from build123d import *
from build123d.topology import SkipClean

# Parameters (mm, degrees)
BOSS_EXTRUDE1_DEPTH = 2
BOSS_EXTRUDE2_START = 3
BOSS_EXTRUDE2_DEPTH = 3
CUT_EXTRUDE1_REACH  = 22.009
SKETCH5_R           = 7.5
BOSS_EXTRUDE3_DEPTH = 1
SKETCH8_W           = 3
SKETCH8_H           = 5
BOSS_EXTRUDE4_DEPTH = 39
BOSS_EXTRUDE5_DEPTH = 2
CUT_EXTRUDE2_REACH  = 72.907
SKETCH10_R          = 3.5
CUT_EXTRUDE4_REACH  = 45.872
SKETCH11_R          = 0.9
BOSS_EXTRUDE6_DEPTH = 7.7
SKETCH16_W          = 2
SKETCH16_H          = 3
BOSS_EXTRUDE7_DEPTH = 14.7


with BuildPart() as part:
    # Sketch2 → Boss-Extrude1 (new body)
    with BuildSketch(Plane.XY):
        with BuildLine():
            ThreePointArc((13.7, 0), (9.687362902, 9.687362902), (0, 13.7))
            ThreePointArc((0, 13.7), (-9.687362902, 9.687362902), (-13.7, 0))
            Line((-13.7, 0), (13.7, 0))
        make_face()
        with BuildLine():
            Line((13.7, 0), (-13.7, 0))
            ThreePointArc((-13.7, 0), (0, -13.7), (13.7, 0))
        make_face()
        with BuildLine():
            Line((13.7, 13.7), (0, 13.7))
            ThreePointArc((0, 13.7), (9.687362902, 9.687362902), (13.7, 0))
            Line((13.7, 0), (13.7, 13.7))
        make_face()
        with BuildLine():
            Line((0, 13.7), (-13.7, 13.7))
            Line((-13.7, 13.7), (-13.7, 0))
            ThreePointArc((-13.7, 0), (-9.687362902, 9.687362902), (0, 13.7))
        make_face()
        with BuildLine():
            ThreePointArc((13.7, 0), (9.687362902, 9.687362902), (0, 13.7))
            ThreePointArc((0, 13.7), (-9.687362902, 9.687362902), (-13.7, 0))
            Line((-13.7, 0), (13.7, 0))
        make_face()
        with BuildLine():
            Line((13.7, 0), (-13.7, 0))
            ThreePointArc((-13.7, 0), (0, -13.7), (13.7, 0))
        make_face()
    extrude(amount=BOSS_EXTRUDE1_DEPTH)

    # Sketch3 → Boss-Extrude2 (add)
    with SkipClean():  # the faces are left unmerged after this step: merging them gives an invalid solid
        with BuildSketch(Plane(origin=(0, 0, 0), x_dir=(-1, 0, 0), z_dir=(0, 0, -1)).offset(BOSS_EXTRUDE2_START)):
            with BuildLine():
                Line((-11.7, 0), (-13.7, 0))
                ThreePointArc((-13.7, 0), (-13.491866216, -2.378980034), (-12.873788905, -4.685675964))
                Line((-12.873788905, -4.685675964), (-10.994403663, -4.001635677))
                ThreePointArc((-10.994403663, -4.001635677), (-11.52225071, -2.031683679), (-11.7, 0))
            make_face()
            with BuildLine():
                ThreePointArc((11.7, 0), (11.52225071, -2.031683679), (10.994403663, -4.001635677))
                Line((10.994403663, -4.001635677), (12.873788905, -4.685675964))
                ThreePointArc((12.873788905, -4.685675964), (13.491866216, -2.378980034), (13.7, 0))
                Line((13.7, 0), (11.7, 0))
            make_face()
        extrude(amount=-BOSS_EXTRUDE2_DEPTH)

    # Sketch5 → Cut-Extrude1 (cut, up to next)
    with BuildSketch(Plane.XY.offset(2), mode=Mode.PRIVATE) as cut_extrude1_sk1:
        Circle(SKETCH5_R)
    cut_extrude1_tool1 = extrude(cut_extrude1_sk1.sketch, amount=-CUT_EXTRUDE1_REACH, mode=Mode.PRIVATE) & part.part
    add(cut_extrude1_tool1.solids().sort_by_distance((0, 0, 2))[0], mode=Mode.SUBTRACT)

    # Sketch7 → Boss-Extrude3 (add)
    with SkipClean():  # the faces are left unmerged after this step: merging them gives an invalid solid
        with BuildSketch(Plane(origin=(0, 13.7, 0), x_dir=(1, 0, 0), z_dir=(0, 1, 0))):
            Polygon((0, 0), (13.7, 0), (0, 27), (-13.7, 0), align=None)
            Polygon((13.7, -2), (13.7, 0), (0, 0), (-13.7, 0), (-13.7, -2), align=None)
        extrude(amount=BOSS_EXTRUDE3_DEPTH)

    # Sketch8 → Boss-Extrude4 (add)
    with SkipClean():  # the faces are left unmerged after this step: merging them gives an invalid solid
        with BuildSketch(Plane.XY.offset(2)):
            with Locations((-12.2, 4.5)):
                Rectangle(SKETCH8_W, SKETCH8_H)
            with Locations((12.2, 4.5)):
                Rectangle(SKETCH8_W, SKETCH8_H)
        extrude(amount=BOSS_EXTRUDE4_DEPTH)

    # Sketch9 → Boss-Extrude5 (add)
    with SkipClean():  # the faces are left unmerged after this step: merging them gives an invalid solid
        with BuildSketch(Plane.XY.offset(41)):
            Polygon((-10.7, 2), (-13.7, 2), (0, -8.786353055), (13.7, 2), (10.7, 2), (10.7, 7), (-10.7, 7), align=None)
        extrude(amount=-BOSS_EXTRUDE5_DEPTH)

    # Sketch10 → Cut-Extrude2 (cut, up to next)
    with BuildSketch(Plane.XY.offset(41), mode=Mode.PRIVATE) as cut_extrude2_sk1:
        Circle(SKETCH10_R)
    cut_extrude2_tool1 = extrude(cut_extrude2_sk1.sketch, amount=-CUT_EXTRUDE2_REACH, mode=Mode.PRIVATE) & part.part
    add(cut_extrude2_tool1.solids().sort_by_distance((0, 0, 41))[0], mode=Mode.SUBTRACT)

    # Sketch11 → Cut-Extrude4 (cut, up to next)
    with BuildSketch(Plane.XY.offset(2), mode=Mode.PRIVATE) as cut_extrude4_sk1:
        with Locations((0, 10)):
            Circle(SKETCH11_R)
    cut_extrude4_tool1 = extrude(cut_extrude4_sk1.sketch, amount=-CUT_EXTRUDE4_REACH, mode=Mode.PRIVATE) & part.part
    # Sketch11 → Cut-Extrude4 (cut, up to next)
    with BuildSketch(Plane.XY.offset(2), mode=Mode.PRIVATE) as cut_extrude4_sk2:
        with Locations((0, -10)):
            Circle(SKETCH11_R)
    cut_extrude4_tool2 = extrude(cut_extrude4_sk2.sketch, amount=-CUT_EXTRUDE4_REACH, mode=Mode.PRIVATE) & part.part
    add(cut_extrude4_tool1.solids().sort_by_distance((0, 10, 2))[0], mode=Mode.SUBTRACT)
    add(cut_extrude4_tool2.solids().sort_by_distance((0, -10, 2))[0], mode=Mode.SUBTRACT)

    # Sketch15 → Boss-Extrude6 (add, through all)
    with SkipClean():  # the faces are left unmerged after this step: merging them gives an invalid solid
        with BuildSketch(Plane(origin=(0, 7, 0), x_dir=(1, 0, 0), z_dir=(0, 1, 0))):
            Polygon((-10.7, -2), (-13.7, -2), (-13.7, -41), (13.7, -41), (13.7, -2), (10.7, -2), (10.7, -39), (-10.7, -39), align=None)
        extrude(amount=BOSS_EXTRUDE6_DEPTH)

    # Sketch16 → Boss-Extrude7 (add, through all)
    with SkipClean():  # the faces are left unmerged after this step: merging them gives an invalid solid
        with BuildSketch(Plane(origin=(0, 0, 0), x_dir=(1, 0, 0), z_dir=(0, 1, 0))):
            with Locations((12.7, 1.5)):
                Rectangle(SKETCH16_W, SKETCH16_H)
            with Locations((-12.7, 1.5)):
                Rectangle(SKETCH16_W, SKETCH16_H)
        extrude(amount=BOSS_EXTRUDE7_DEPTH)


solid = part.part
Input: part model. Units: mm. Frame: model coordinates. A direction names the side the tool comes from. Round coordinates to 2 decimals unless told otherwise and drop trailing zeros. Loops run counter-clockwise (first coordinate to the right, second up) from the corner with the lowest first, then second, coordinate; pieces in that order, holes last. Notation, with made-up numbers: (80.5, 53.25) -> (118.5, 53.25) arc R17 ccw to (118.5, 63.25) -> close; hole circle Ø5 at (-32, -5). An arc over 180 degrees is marked (long way). Answer as a JSON object with one key per item and string values. Group by question number.
1) Section query B-B on z = 1. Output: boundary loops of the cut face in (x, y).
2) Ray query, L1, parallel to Y at x = 0, z = 1.65; L2, parallel to Z at x = 9.25, y = 7.25; L3, parallel to X at y = 2.25, z = 24. Return the intervals inside material, ascending.
3) Section query C-C on y = 10. Output: boundary loops of the cut face in (x, z), plus the area to 3 significant figures.
4) Section query A-A on z = 21.5. Output: boundary loops of the cut face in (x, y).
5) Section query D-D on x = 5.25. Output: boundary loops of the cut face in (y, z).
6) Draft query along Z for faces 1 (the cylindrical face through (-7.493, 0.33, 1.014)), 2 (the flat face through (-10.7, 8, 20)), 3 (the flat face through (6.174, 14.193, -14.832)). Return one class per face: +Z half, -Z half, draft (parallel to the pull), parting line (faces both ways), or undercut.
7) Reachability of faces 4 (the flat face through (10.7, 8, 20)), 5 (the flat face through (12, 2, 20)), 6 (the flat face through (-11.7, 7, -1)) from +Z, -Z, +X, -X, +Y, -Y: full face, straight path, thin tool, end or side. Return the list, or none.
8) Pin query (flat end, axial travel): pin 1 (4 mm diameter, centred on x = -4.5, y = 0, fed in from -Z); pin 2 (1.4 mm diameter, centred on x = -12, y = 6, fed in from -Z); pin 3 (3.5 mm diameter, centred on x = -12, z = 12, fed in from -Y). Return the tip coordinate at first contact, or that it passes through.
Reply:
{
 "1": {"outline": "(-13.7, 0) arc R13.7 ccw to (13.7, 0) -> (13.7, 14.7) -> (-13.7, 14.7) -> close; hole circle Ø15 at (0, 0); hole circle Ø1.8 at (0, -10); hole circle Ø1.8 at (0, 10)"},
 "2": {"L1": "y = -13.7 to -10.9, -9.1 to -7.5, 7.5 to 9.1, 10.9 to 14.7", "L2": "z = 0 to 2, 39 to 41", "L3": "x = -13.7 to -10.7, 10.7 to 13.7"},
 "3": {"outline": "(-13.7, -3) -> (-11.7, -3) -> (-11.7, 0) -> (-0.9, 0) -> (-0.9, 2) -> (-10.7, 2) -> (-10.7, 39) -> (10.7, 39) -> (10.7, 2) -> (0.9, 2) -> (0.9, 0) -> (11.7, 0) -> (11.7, -3) -> (13.7, -3) -> (13.7, 41) -> (-13.7, 41) -> close", "area": "340 mm2"},
 "4": {"outline": "(-13.7, 2) -> (-10.7, 2) -> (-10.7, 14.7) -> (-13.7, 14.7) -> close; (10.7, 2) -> (13.7, 2) -> (13.7, 14.7) -> (10.7, 14.7) -> close"},
 "5": {"outline": "(-12.65, 0) -> (-5.36, 0) -> (-5.36, 2) -> (-12.65, 2) -> close; (-4.65, 39) -> (14.7, 39) -> (14.7, 41) -> (-4.65, 41) -> close; (5.36, 0) -> (13.7, 0) -> (13.7, -16.65) -> (14.7, -16.65) -> (14.7, 2) -> (5.36, 2) -> close"},
 "6": {"face 1": "draft", "face 2": "undercut", "face 3": "-Z half"},
 "7": {"face 4": "+Y, -Y", "face 5": "+X, -X, -Y", "face 6": "-Z"},
 "8": {"pin 1": "stops at z = 39", "pin 2": "stops at z = -3", "pin 3": "stops at y = 2"}
}
